Here's the drawing with two shaded views (mm, measured from the low corner). I have some questions. A direction names the side the tool comes from. Coordinates: 2 decimals unless noted, no trailing zeros. Write each loop counter-clockwise with the first axis right and the second up, starting at its lowest first coordinate (ties: lowest second). Pieces come first, ordered by that corner, then holes.
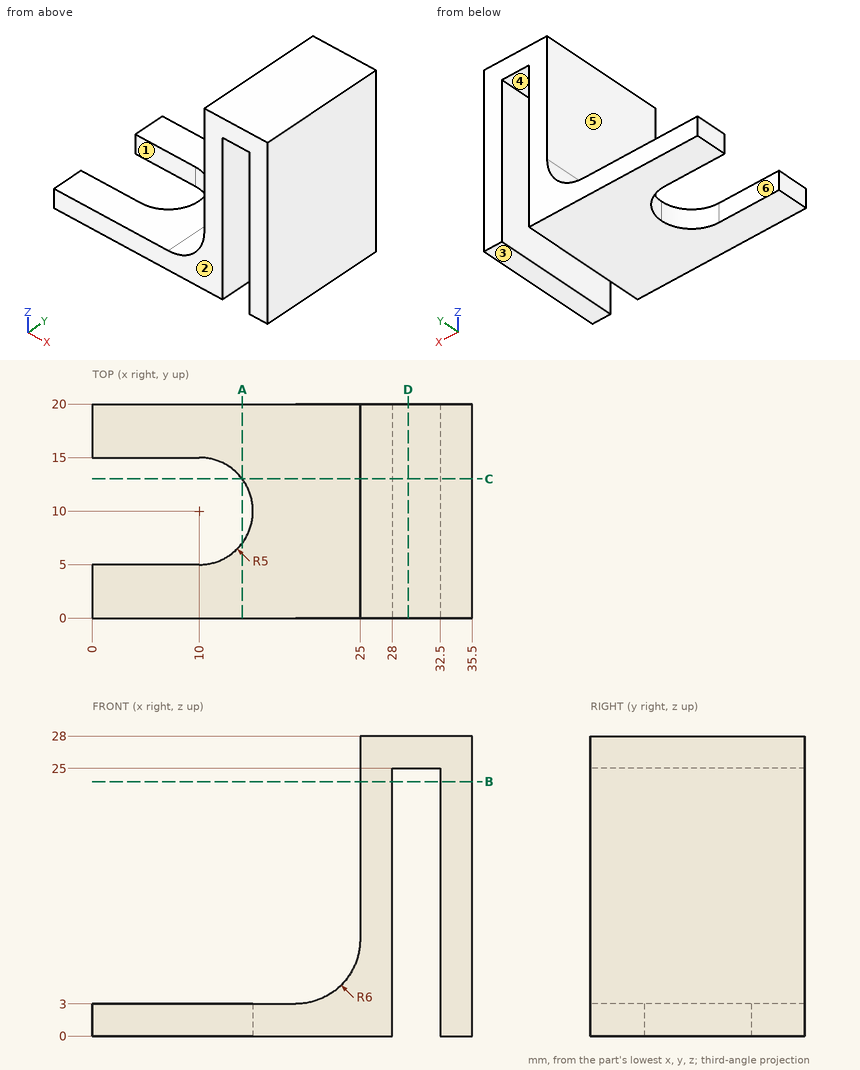
Item 1: I want a section at A-A, the plane x = 14. List the corners of the cut face in (y, z) for me, then the cut area to 3 significant figures.
Item 2: If I drill on line 1 along X through (y, z) = (7.5, 24.25); line 2 along X through (y, z) = (15.25, 2.25); line 3 along Z through (x, y) = (32, 14), over which ranges is the centre line in solid material (lowest first)?
Item 3: I want a section at D-D, the plane x = 29.5. List the corners of the cut face in (y, z) for me, then the cut area to 3 significant figures.
Item 4: I want a section at C-C, the plane y = 13. List the corners of the cut face in (x, z) for me.
Item 5: Which directions (+Z, -Z, +X, -X, +Y, -Y) give clear straight access to the entire face, cutting with the end or side of a thin tool? Please do the marked faces 4, 5 and 6.
Item 6: If we mould it in two halves opening along Y, with no side actions, what happens to the marked faces 1, 2 and 3? For each: released by +Y, released by -Y, zero draft, split by the parting line, or undercut.
Item 7: I want a section at B-B, the plane z = 23.75. List the corners of the cut face in (x, y) for me.
Taken from the geometry:
1. outline: (0, 0) - (7, 0) - (7, 3) - (0, 3) - close; (13, 0) - (20, 0) - (20, 3) - (13, 3) - close
1. area: 42.0 mm2
2. line 1: x = 25 to 28, 32.5 to 35.5
2. line 2: x = 0 to 28, 32.5 to 35.5
2. line 3: z = 25 to 28
3. outline: (0, 25) - (20, 25) - (20, 28) - (0, 28) - close
3. area: 60.0 mm2
4. outline: (14, 0) - (28, 0) - (28, 25) - (32.5, 25) - (32.5, 0) - (35.5, 0) - (35.5, 28) - (25, 28) - (25, 9) arc R6 cw to (19, 3) - (14, 3) - close
5. face 4: -Z, +Y, -Y
5. face 5: +Z, -X, +Y, -Y
5. face 6: +Z, -Z, -X
6. face 1: undercut
6. face 2: released by -Y
6. face 3: zero draft
7. outline: (25, 0) - (28, 0) - (28, 20) - (25, 20) - close; (32.5, 0) - (35.5, 0) - (35.5, 20) - (32.5, 20) - close
